```python
from build123d import *

# Parameters (mm, degrees)
EXTRUDE_1_DEPTH     = 1
SKETCH_4_W          = 197
SKETCH_4_H          = 140
CUT_EXTRUDE_3_DEPTH = 0.5


with BuildPart() as part:
    # 草图1 → 凸台-拉伸1 (new body)
    with BuildSketch(Plane(origin=(0, 0, 0), x_dir=(1, 0, 0), z_dir=(0, 1, 0))):
        Polygon((-98.5, 60), (-100.5, 60), (-100.5, -60), (-98.5, -60), (-98.5, -70), (98.5, -70), (98.5, -60), (100.5, -60), (100.5, 60), (98.5, 60), (98.5, 70), (-98.5, 70), align=None)
    extrude(amount=EXTRUDE_1_DEPTH)

    # 草图4 → 切除-拉伸3 (cut)
    with BuildSketch(Plane(origin=(0, 0, 0), x_dir=(1, 0, 0), z_dir=(0, 1, 0))):
        Rectangle(SKETCH_4_W, SKETCH_4_H)
    extrude(amount=CUT_EXTRUDE_3_DEPTH, mode=Mode.SUBTRACT)


solid = part.part
```
Can you work these out from the model? Positions are in its coordinate system, mm. Coordinates: 2 decimals unless noted, no trailing zeros. Write each loop counter-clockwise with the first axis right and the second up, starting at its lowest first coordinate (ties: lowest second). Pieces come first, ordered by that corner, then holes. Notation, with made-up numbers: M 14,14.5 L 36,14.5 A4 ccw 36,19.5 Z; hole C 28.5,-32.5 d2. An arc over 180 degrees is marked long. Write item = value, one per line. Start each with the question number.
Q1. If we section it at B-B, the plane x = 68.5: Write out the boundary of the cut face in (y, z), then the cut area to 3 significant figures.
Q2. If we section it at A-A, the plane z = -49: Write out the boundary of the cut face in (x, y).
Q3. If I drill on L1, parallel to X at y = 0.4, z = 12; L2, parallel to Y at x = 64, z = -61.5, over which ranges is the centre line in solid material (lowest first)? Write a range as [from, to].
Q4. I'm going to push flat-ended pins straight in: pin 1 (0.5 mm diameter, centred on x = 100, y = 0.5, fed in from +Z); pin 2 (0.5 mm diameter, centred on x = 100, y = 0.5, fed in from -Z); pin 3 (5 mm diameter, centred on x = -35, z = -33, fed in from -Y). Where does each tip first touch, or does it pass through?
Q5. Thinking about a two-plate mould opening in X: for faces 1 (the face through (-1, 0.5, -1)), 2 (the face through (-1, 1, -1)), which applies, released by +X, released by -X, zero draft, split by the parting line, or undercut?
Check sheet entries:
q1.outline = M 0.5,-70 L 1,-70 L 1,70 L 0.5,70 Z
q1.area = 70.0 mm²
q2.outline = M -100.5,0 L -98.5,0 L -98.5,0.5 L 98.5,0.5 L 98.5,0 L 100.5,0 L 100.5,1 L -100.5,1 Z
q3.L1 = [-100.5, -98.5], [98.5, 100.5]
q3.L2 = [0.5, 1]
q4.pin_1 = 60
q4.pin_2 = -60
q4.pin_3 = 0.5
q5.face_1 = undercut
q5.face_2 = zero draft
